CAD build for the part. Positions are in the model's coordinates, mm. Coordinates: 2 decimals unless noted, no trailing zeros. Order: outer loops, then holes, each group sorted by start corner. A loop starts at its lowest first (then second) coordinate and runs counter-clockwise, first axis right, second up.
from build123d import *

# Parameters (mm, degrees)
SKETCH1_R           = 2.0193
BOSS_EXTRUDE1_DEPTH = 3.175


with BuildPart() as part:
    # Sketch1 → Boss-Extrude1 (new body)
    with BuildSketch(Plane.XY):
        Polygon((0, 114.3), (88.9, 114.3), (88.9, 0), (215.9, 0), (215.9, 114.3), (304.8, 114.3), (304.8, 279.4), (0, 279.4), align=None)
        with Locations((101.6, 12.7)):
            Circle(SKETCH1_R, mode=Mode.SUBTRACT)
        with Locations((114.3, 12.7)):
            Circle(SKETCH1_R, mode=Mode.SUBTRACT)
        with Locations((127, 12.7)):
            Circle(SKETCH1_R, mode=Mode.SUBTRACT)
        with Locations((139.7, 12.7)):
            Circle(SKETCH1_R, mode=Mode.SUBTRACT)
        with Locations((12.7, 127)):
            Circle(SKETCH1_R, mode=Mode.SUBTRACT)
        with Locations((12.7, 139.7)):
            Circle(SKETCH1_R, mode=Mode.SUBTRACT)
        with Locations((12.7, 152.4)):
            Circle(SKETCH1_R, mode=Mode.SUBTRACT)
        with Locations((12.7, 165.1)):
            Circle(SKETCH1_R, mode=Mode.SUBTRACT)
        with Locations((12.7, 177.8)):
            Circle(SKETCH1_R, mode=Mode.SUBTRACT)
        with Locations((12.7, 190.5)):
            Circle(SKETCH1_R, mode=Mode.SUBTRACT)
        with Locations((12.7, 203.2)):
            Circle(SKETCH1_R, mode=Mode.SUBTRACT)
        with Locations((12.7, 215.9)):
            Circle(SKETCH1_R, mode=Mode.SUBTRACT)
        with Locations((12.7, 228.6)):
            Circle(SKETCH1_R, mode=Mode.SUBTRACT)
        with Locations((12.7, 241.3)):
            Circle(SKETCH1_R, mode=Mode.SUBTRACT)
        with Locations((12.7, 254)):
            Circle(SKETCH1_R, mode=Mode.SUBTRACT)
        with Locations((12.7, 266.7)):
            Circle(SKETCH1_R, mode=Mode.SUBTRACT)
        with Locations((292.1, 266.7)):
            Circle(SKETCH1_R, mode=Mode.SUBTRACT)
        with Locations((292.1, 254)):
            Circle(SKETCH1_R, mode=Mode.SUBTRACT)
        with Locations((292.1, 241.3)):
            Circle(SKETCH1_R, mode=Mode.SUBTRACT)
        with Locations((292.1, 228.6)):
            Circle(SKETCH1_R, mode=Mode.SUBTRACT)
        with Locations((292.1, 215.9)):
            Circle(SKETCH1_R, mode=Mode.SUBTRACT)
        with Locations((292.1, 203.2)):
            Circle(SKETCH1_R, mode=Mode.SUBTRACT)
        with Locations((292.1, 190.5)):
            Circle(SKETCH1_R, mode=Mode.SUBTRACT)
        with Locations((292.1, 177.8)):
            Circle(SKETCH1_R, mode=Mode.SUBTRACT)
        with Locations((292.1, 165.1)):
            Circle(SKETCH1_R, mode=Mode.SUBTRACT)
        with Locations((292.1, 152.4)):
            Circle(SKETCH1_R, mode=Mode.SUBTRACT)
        with Locations((292.1, 139.7)):
            Circle(SKETCH1_R, mode=Mode.SUBTRACT)
        with Locations((292.1, 127)):
            Circle(SKETCH1_R, mode=Mode.SUBTRACT)
        with Locations((165.1, 12.7)):
            Circle(SKETCH1_R, mode=Mode.SUBTRACT)
        with Locations((177.8, 12.7)):
            Circle(SKETCH1_R, mode=Mode.SUBTRACT)
        with Locations((190.5, 12.7)):
            Circle(SKETCH1_R, mode=Mode.SUBTRACT)
        with Locations((203.2, 12.7)):
            Circle(SKETCH1_R, mode=Mode.SUBTRACT)
    extrude(amount=BOSS_EXTRUDE1_DEPTH)


solid = part.part
1) Slice it at C-C (x = 240). List the corners of the cut face in (y, z) (3 decimals), plus the area to 3 significant figures.
2) Slice it at A-A (z = 0.7). Give the number of separate pieces and of enclosed holes in the cut face, plus the area to 3 significant figures.
3) Drill centre lines: probe 1 along X at (y, z) = (165.1, 1.2); probe 2 along Y at (x, z) = (203.2, 2.05); probe 3 along X at (y, z) = (53, 2.7). Where is each one in solid material? Low to high.
4) Slice it at B-B (y = 69.5). List the corners of the cut face in (x, z) (3 decimals).
Worked out:
1. outline: (114.3, 0) - (279.4, 0) - (279.4, 3.175) - (114.3, 3.175) - close
1. area: 524 mm2
2. separate pieces: 1
2. enclosed holes: 32
2. area: 64,400 mm2
3. probe 1: x = 0 to 10.68, 14.72 to 290.08, 294.12 to 304.8
3. probe 2: y = 0 to 10.68, 14.72 to 279.4
3. probe 3: x = 88.9 to 215.9
4. outline: (88.9, 0) - (215.9, 0) - (215.9, 3.175) - (88.9, 3.175) - close
